Build history of the part. All positions in model axes, mm. A direction names the side the tool comes from. Give positions to 0.01 mm unless a question says otherwise; leave off trailing zeros. Loops run counter-clockwise (first coordinate to the right, second up) from the corner with the lowest first, then second, coordinate; pieces in that order, holes last.
1) Band-saw the part on B-B on z = 0. List the corners of the cut face in (x, y) (3 decimals).
2) Band-saw the part on A-A on x = 0. List the corners of the cut face in (y, z) (3 decimals).
3) Wall check: line 1 (Y direction, x = 0.5, z = -2.75); line 2 (Z direction, x = -0.25, y = 7.5); line 3 (X direction, y = -19, z = 2). Give the ranges that are in metal, low to high.
4) Flat gauge pins, fed straight in: P1, Ø3, axis at x = -2, y = 1.5, coming from the -Z side; P2, Ø1, axis at y = 22, z = 1.5, coming from the +X side; P3, Ø1, axis at y = -12.5, z = -2.5, coming from the -X side. Where does each tip first touch, or does it go through?
5) 3-axis set-ups, long thin cutter, end or side, ignore diameter. For faces 1 (the cylindrical face through (-1.468, -27.14, -1.915)), 2 (the cylindrical face through (-1.468, 27.14, -1.915)), 3 (the flat face through (0, -33.401, 0)): which of +Z, -Z, +X, -X, +Y, -Y reach the whole face in a straight line?
6) Band-saw the part on C-C on y = -5. List the corners of the cut face in (x, z) (3 decimals), then the cut area to 3 significant figures.
```python
from build123d import *

# Parameters (mm, degrees)
SKETCH2_R           = 3.175
BOSS_EXTRUDE1_DEPTH = 20.701
SKETCH3_R           = 2.413
BOSS_EXTRUDE2_DEPTH = 12.7


with BuildPart() as part:
    # Sketch2 → Boss-Extrude1 (new, symmetric)
    with BuildSketch(Plane(origin=(0, 0, 0), x_dir=(1, 0, 0), z_dir=(0, 1, 0))):
        with Locations(Location((0, 0, 0), (0, 0, 270))):
            Circle(SKETCH2_R)
    extrude(amount=BOSS_EXTRUDE1_DEPTH, both=True)

    # Sketch3 → Boss-Extrude2 (add, symmetric)
    with BuildSketch(Plane(origin=(0, 20.701, 0), x_dir=(1, 0, 0), z_dir=(0, 1, 0))):
        with Locations(Location((0, 0, 0), (0, 0, 270))):
            Circle(SKETCH3_R)
    boss_extrude2 = extrude(amount=BOSS_EXTRUDE2_DEPTH, both=True)

    # Mirror1: Boss-Extrude2 across plane
    add(boss_extrude2.mirror(Plane.ZX))


solid = part.part
```
Findings below:
1. outline: (-3.175, -20.701) - (-2.413, -20.701) - (-2.413, -33.401) - (2.413, -33.401) - (2.413, -20.701) - (3.175, -20.701) - (3.175, 20.701) - (2.413, 20.701) - (2.413, 33.401) - (-2.413, 33.401) - (-2.413, 20.701) - (-3.175, 20.701) - close
2. outline: (-33.401, -2.413) - (-20.701, -2.413) - (-20.701, -3.175) - (20.701, -3.175) - (20.701, -2.413) - (33.401, -2.413) - (33.401, 2.413) - (20.701, 2.413) - (20.701, 3.175) - (-20.701, 3.175) - (-20.701, 2.413) - (-33.401, 2.413) - close
3. line 1: y = -20.7 to 20.7
3. line 2: z = -3.17 to 3.17
3. line 3: x = -2.47 to 2.47
4. P1: stops at z = -3.14
4. P2: stops at x = 2.2
4. P3: stops at x = -2.47
5. face 1: -Y
5. face 2: +Y
5. face 3: +Z, -Z, +X, -X, -Y
6. outline: circle Ø6.35 at (0, 0)
6. area: 31.7 mm2
